Autodesk Inventor part; units mm, degrees
ref_plane "YZ Plane" through (0, 0, 0) normal (1, 0, 0) x (0, 1, 0)
ref_plane "XZ Plane" through (0, 0, 0) normal (0, 1, 0) x (-1, 0, 0)
ref_plane "XY Plane" through (0, 0, 0) normal (0, 0, 1) x (1, 0, 0)
sketch "Sketch1" plane through (0, 0, 0) normal (0, 1, 0) x (-1, 0, 0)
  circle A0 centre (0, 0) radius 3.5
  dimension "d0" = 7
extrude "Extrusion1" add sketch "Sketch1" along normal blind 17
sketch "Sketch2" plane through (0, 17, 0) normal (0, 1, 0) x (1, 0, 0)
  circle A0 centre (0, 0) radius 0.5
  dimension "d3" = 1
extrude "Extrusion2" add sketch "Sketch2" along normal blind 5
sketch "Sketch3" plane through (0, 22, 0) normal (0, 1, 0) x (1, 0, 0)
  circle A0 centre (0, 0) radius 0.5
  line L0 (-0.0995, 0.49) -> (0.0995, 0.49)
  circle A1 centre (0, 0) radius 0.5
  line L1 (0.4999, 0.0075) -> (0.4999, 0.0075)
  line L2 (0.49, 0.0995) -> (0.49, -0.0995)
  dimension "d8" = 0.49
  dimension "d9" = 0.49
extrude "Extrusion3" cut sketch "Sketch3" against normal blind 0.1 contours A0 L2 | L0 A0
properties part number "motor" material "Steel"
The model under review builds one solid part; all positions refer to its coordinate system, in mm. A direction names the side the tool comes from. Give positions to 0.01 mm unless a question says otherwise; leave off trailing zeros. Order: outer loops, then holes, each group sorted by start corner. A loop starts at its lowest first (then second) coordinate and runs counter-clockwise, first axis right, second up. Notation, with made-up numbers: M 45.5,5 L 94.5,5 A32 ccw 94.5,43 Z; hole C 65.25,80.25 d5. An arc over 180 degrees is marked long. Answer in a Markdown table with one row per item. Add a question column.
1. Add section A-A on y = 3.75. State the section outline as (x, z) points, plus the area to 3 significant figures.
2. To check wall thickness, follow line 1 along Y through (x, z) = (1, 1); line 2 along X through (y, z) = (8, -3); line 3 along Z through (x, y) = (-0.75, 9.5). State the ranges of each line that lie inside material, in increasing order.
3. For pin 1 Ø2 at (x, z) = (-1, 1) entering from +Y; pin 2 Ø3 at (x, z) = (-2.5, 0) entering from +Y; pin 3 Ø2 at (y, z) = (10.5, -2.5) entering from +X; pin 4 Ø4 at (y, z) = (4, -2.5) entering from -X, all flat-tipped, find the tip position at first contact; note any pin that passes through.
4. Add section D-D on y = 18.5. State the section outline as (x, z) points.
5. Add section B-B on x = -2. State the section outline as (y, z) points, plus the area to 3 significant figures.
6. Machinability: for faces 1 (the cylindrical face through (-0.108, 19.465, -0.488)), 2 (the flat face through (0, 22, 0)), which of the approach directions +Z, -Z, +X, -X, +Y, -Y give a long, thin tool a straight path to every point of the face, cutting with its end or side? Answer none if there is none.
7. Add section C-C on z = 1.5. State the section outline as (x, y) points, plus the area to 3 significant figures.
The answers:
| question | item | result |
|---|---|---|
| 1 | outline | C 0,0 d7 |
| 1 | area | 38.5 mm2 |
| 2 | line 1 | 0 to 17 |
| 2 | line 2 | -1.8 to 1.8 |
| 2 | line 3 | -3.42 to 3.42 |
| 3 | pin 1 | y = 22 |
| 3 | pin 2 | y = 17 |
| 3 | pin 3 | x = 3.16 |
| 3 | pin 4 | x = -3.46 |
| 4 | outline | C 0,0 d1 |
| 5 | outline | M 0,-2.87 L 17,-2.87 L 17,2.87 L 0,2.87 Z |
| 5 | area | 97.7 mm2 |
| 6 | face 1 | +Y |
| 6 | face 2 | +Z, -Z, +X, -X, +Y |
| 7 | outline | M -3.16,0 L 3.16,0 L 3.16,17 L -3.16,17 Z |
| 7 | area | 108 mm2 |
